Autodesk Inventor part; units mm, degrees
ref_plane "YZ Plane" through (0, 0, 0) normal (1, 0, 0) x (0, 1, 0)
ref_plane "XZ Plane" through (0, 0, 0) normal (0, 1, 0) x (-1, 0, 0)
ref_plane "XY Plane" through (0, 0, 0) normal (0, 0, 1) x (1, 0, 0)
sketch "Sketch5" plane through (0, 0, 0) normal (0, 1, 0) x (-1, 0, 0)
  circle A0 centre (0, 0) radius 2.55
  circle A1 centre (0, 0) radius 7.5
  circle A2 centre (0, 0) radius 36
  dimension "d10" = 5.1
  dimension "d11" = 15
  dimension "d12" = 72
extrude "Extrusion4" add sketch "Sketch5" along normal blind 10 contours A2
extrude "Extrusion5" add sketch "Sketch5" along normal blind 15 contours A1
sketch "Sketch6" plane through (0, 0, 0) normal (0, -1, 0) x (1, 0, 0)
  circle A0 centre (0, 0) radius 10
  circle A1 centre (0, 0) radius 2.55
  circle A2 centre (0, 0) radius 36
  circle A3 centre (0, 0) radius 2.55
  circle A4 centre (0, 0) radius 31
  line L0 (-30.5941, 5) -> (-10, 5)
  line L1 (-30.5941, -5) -> (-10, -5)
  line L2 (-10, -5) -> (-8.6603, -5)
  line L3 (-10, 5) -> (-8.6603, 5)
  circle A5 centre (0, 0) radius 10
  line L4 (8.6603, -5) -> (30.5941, -5)
  line L5 (8.6603, 5) -> (30.5941, 5)
  line L6 (5, 10) -> (5, 30.5941)
  line L7 (5, 10) -> (5, 8.6603)
  line L8 (5, -8.6603) -> (5, -30.5941)
  line L9 (-5, 8.6603) -> (-5, 30.5941)
  line L10 (-5, -8.6603) -> (-5, -30.5941)
  dimension "d17" = 20
extrude "Extrusion6" cut sketch "Sketch6" against normal up to surface (10 mm away) contours A0 L7 L6 A4 L5 | L4 A4 L8 A0 | A0 L3 L0 A4 L9 | L10 A4 L1 L2 A0
fillet "Fillet1" radius 2 8 edges at (-5, 5, -30.5941) (-30.5941, 5, -5) (-30.5941, 5, 5) (-5, 5, 30.5941) (5, 5, 30.5941) (30.5941, 5, 5) (30.5941, 5, -5) (5, 5, -30.5941)
fillet "Fillet2" radius 2 1 edges at (7.5, 10, 0)
properties part number "wheel"
Work out the finished part from the listing and answer in its coordinate system (mm). Coordinates: 2 decimals unless noted, no trailing zeros. Loops run counter-clockwise (first coordinate to the right, second up) from the corner with the lowest first, then second, coordinate; pieces in that order, holes last. Notation, with made-up numbers: (18.25, 56) -> (75.25, 56) arc R23 cw to (75.25, 92) -> close; hole circle Ø10 at (21, 13). An arc over 180 degrees is marked (long way). Answer as CSV lines item,"result".
1) For a pull along Z with two mould halves and no side action, classify faces 1 (the face through (8.2, 10, -5.2)), 2 (the face through (-5, 5, 18)) as released by +Z, released by -Z, zero draft, split by the parting line, or undercut.
A:
face 1,"zero draft"
face 2,"undercut"
2) The part is cut by section A-A (x = 0). Give the vertices of the cut face in (y, z).
A:
outline,"(0, -36) -> (10, -36) -> (10, -9.5) arc R2 cw to (12, -7.5) -> (15, -7.5) -> (15, -2.55) -> (0, -2.55) -> close; (0, 2.55) -> (15, 2.55) -> (15, 7.5) -> (12, 7.5) arc R2 cw to (10, 9.5) -> (10, 36) -> (0, 36) -> close"
3) The part is cut by section C-C (z = 29). Give the vertices of the cut face in (x, y).
A:
outline,"(-21.33, 0) -> (-10.95, 0) -> (-10.95, 10) -> (-21.33, 10) -> close; (-5.19, 0) -> (5.19, 0) -> (5.19, 10) -> (-5.19, 10) -> close; (10.95, 0) -> (21.33, 0) -> (21.33, 10) -> (10.95, 10) -> close"
4) The part is cut by section B-B (z = 0). Give the vertices of the cut face in (x, y), and give its area (3 significant figures).
A:
outline,"(-36, 0) -> (-2.55, 0) -> (-2.55, 15) -> (-7.5, 15) -> (-7.5, 12) arc R2 cw to (-9.5, 10) -> (-36, 10) -> close; (2.55, 0) -> (36, 0) -> (36, 10) -> (9.5, 10) arc R2 cw to (7.5, 12) -> (7.5, 15) -> (2.55, 15) -> close"
area,"720 mm²"
5) Flat-ended cylindrical pins translate along their axes: pin 1 (8 mm diameter, centred on x = 11.5, y = 7.5, fed in from +Z); pin 2 (2 mm diameter, centred on y = 4.5, z = -13, fed in from +X); pin 3 (1.5 mm diameter, centred on x = 17.5, y = 7, fed in from +Z); pin 4 (4 mm diameter, centred on x = 0, z = 0, fed in from -Y). Find the tip coordinate at first contact, or state that the pin passes through.
A:
pin 1,"stops at z = 35.21"
pin 2,"stops at x = 33.94"
pin 3,"stops at z = 31.87"
pin 4,"passes through"
6) Straight lines are drawn through the part: probe 1 along Z at (x, y) = (0, 9); probe 2 along Z at (x, y) = (7.5, 5.25); probe 3 along Z at (x, y) = (0, 12). For each, find the intervals that lie inside material, in ascending order.
A:
probe 1,"z = -36 to -2.55, 2.55 to 36"
probe 2,"z = -35.21 to -30.08, -6.61 to 6.61, 30.08 to 35.21"
probe 3,"z = -7.5 to -2.55, 2.55 to 7.5"
7) The part is cut by section D-D (y = 9). Give the vertices of the cut face in (x, z).
A:
outline,"circle Ø72 at (0, 0); hole (-30.08, -7.48) arc R31 ccw to (-7.48, -30.08) arc R2 ccw to (-5, -28.14) -> (-5, -8.66) arc R10 cw to (-8.66, -5) -> (-28.14, -5) arc R2 ccw to start; hole (-30.08, 7.48) arc R2 ccw to (-28.14, 5) -> (-8.66, 5) arc R10 cw to (-5, 8.66) -> (-5, 28.14) arc R2 ccw to (-7.48, 30.08) arc R31 ccw to start; hole circle Ø5.1 at (0, 0); hole (5, -28.14) arc R2 ccw to (7.48, -30.08) arc R31 ccw to (30.08, -7.48) arc R2 ccw to (28.14, -5) -> (8.66, -5) arc R10 cw to (5, -8.66) -> close; hole (5, 8.66) arc R10 cw to (8.66, 5) -> (28.14, 5) arc R2 ccw to (30.08, 7.48) arc R31 ccw to (7.48, 30.08) arc R2 ccw to (5, 28.14) -> close"
